```python
from build123d import *

# Parameters (mm, degrees)
F2_DEPTH = 38.1
F3_DEPTH = 50.8


with BuildPart() as f2:
    # F1 (on Top) → F2 (new body)
    with BuildSketch(Plane.XY):
        Polygon((24.104279, 0), (46.047091, 0), (46.047091, 10.441257), (35.075685, 10.441257), (35.075685, 27.602856), (46.047091, 27.602856), (46.047091, 38.044113), (24.104279, 38.044113), align=None)
        Polygon((10.73552, 0), (24.104279, 0), (24.104279, 38.044113), (10.73552, 38.044113), (10.73552, 27.602856), (0, 27.602856), (0, 10.441257), (10.73552, 10.441257), align=None)
    extrude(amount=F2_DEPTH)

    # F0 (on Front) → F3 (cut)
    with BuildSketch(Plane.XZ):
        Polygon((24.104279, 43.043356), (46.047091, 25.215129), (46.047091, 43.043356), align=None)
    extrude(amount=-F3_DEPTH, mode=Mode.SUBTRACT)


solid = f2.part
```
Design review of the part built by this model. Coordinates are the model's own, in mm. A direction names the side the tool comes from. Round coordinates to 2 decimals unless told otherwise and drop trailing zeros. Order: outer loops, then holes, each group sorted by start corner. A loop starts at its lowest first (then second) coordinate and runs counter-clockwise, first axis right, second up. Notation, with made-up numbers: M 71,10.5 L 129,10.5 A22 cw 129,30.5 Z; hole C -20.5,64.5 d6. An arc over 180 degrees is marked long. Put each result on its own line as item: value.
Q1. Draft analysis for pull direction Y (two halves, no side actions). For faces 5 (the face through (5, 10.441, 19)), 6 (the face through (35.076, 19, 17)), 7 (the face through (0, 19, 19)), state which applies: released by +Y, released by -Y, zero draft, split by the parting line, or undercut.
Reported:
face 5: released by -Y
face 6: undercut
face 7: zero draft
Q2. To check wall thickness, follow line 1 (Y direction, x = 39.5, z = 3.5); line 2 (Y direction, x = 9, z = 15); line 3 (X direction, y = 29.5, z = 13.5). State the ranges of each line that lie inside material, in increasing order.
Reported:
line 1: 0 to 10.44, 27.6 to 38.04
line 2: 10.44 to 27.6
line 3: 10.74 to 46.05
Q3. Machinability: for faces 1 (the face through (18, 19, 38.1)), 2 (the face through (10.736, 5, 19)), 3 (the face through (10.736, 33, 19)), 4 (the face through (41, 10.441, 13)), which of the approach directions +Z, -Z, +X, -X, +Y, -Y give a long, thin tool a straight path to every point of the face, cutting with its end or side? Answer none if there is none.
Reported:
face 1: +Z, +X, -X, +Y, -Y
face 2: +Z, -Z, -X, -Y
face 3: +Z, -Z, -X, +Y
face 4: +Z, -Z, +X
Q4. Insertion check: pin 1 Ø8.5 at (y, z) = (6, 11) entering from -X; pin 2 Ø3.5 at (x, z) = (41, 21) entering from -Y; pin 3 Ø12 at (x, z) = (4.5, 17.5) entering from +Y; pin 4 Ø12 at (x, z) = (3, 26) entering from -Y. Each pin has a flat end and moves straight along its axis. Give the tip position at first contact, or say it passes through.
Reported:
pin 1: x = 10.74
pin 2: y = 0
pin 3: y = 27.6
pin 4: y = 10.44
Q5. Consider section A-A (y = 25). State the section outline as (x, z) points, and give its area (3 significant figures).
Reported:
outline: M 0,0 L 35.08,0 L 35.08,34.13 L 30.19,38.1 L 0,38.1 Z
area: 1,330 mm²
Q6. Consider section B-B (z = 16). State the section outline as (x, y) points, and give its area (3 significant figures).
Reported:
outline: M 0,10.44 L 10.74,10.44 L 10.74,0 L 46.05,0 L 46.05,10.44 L 35.08,10.44 L 35.08,27.6 L 46.05,27.6 L 46.05,38.04 L 10.74,38.04 L 10.74,27.6 L 0,27.6 Z
area: 1,340 mm²
Q7. Consider section D-D (y = 36). State the section outline as (x, z) points, and give its area (3 significant figures).
Reported:
outline: M 10.74,0 L 46.05,0 L 46.05,25.22 L 30.19,38.1 L 10.74,38.1 Z
area: 1,240 mm²
Q8. Consider section C-C (x = 5.5). State the section outline as (y, z) points, and give its area (3 significant figures).
Reported:
outline: M 10.44,0 L 27.6,0 L 27.6,38.1 L 10.44,38.1 Z
area: 654 mm²
